Geometry: see drawing. Coordinates: mm, zero at the bounding-box minimum. A direction names the side the tool comes from. Give positions to 0.01 mm unless a question says otherwise; leave off trailing zeros. Write each loop counter-clockwise with the first axis right and the second up, starting at its lowest first coordinate (ties: lowest second). Pieces come first, ordered by that corner, then holes. Notation, with made-up numbers: (-24, 48) -> (2, 48) arc R23 ccw to (2, 56) -> close; hole circle Ø9 at (77.25, 58.25). An arc over 180 degrees is marked (long way). Use one line per item in the form item = value. Start each with the question number.
(1) Cut plane A-A, the plane y = 63.5. Output: boundary loops of the cut face in (x, z) (1 decimal).
(2) Material intervals for line 1 along X through (y, z) = (114, 19); line 2 along Y through (x, z) = (13, 23.5); line 3 along Z through (x, y) = (37, 121.5), sorted ascending. Write a range as from..to.
(3) Cut plane B-B, the plane z = 9. Output: boundary loops of the cut face in (x, y), and give its area (3 significant figures).
(4) Set-up query: the marked faces 1 and 2. Return all of +Z, -Z, +X, -X, +Y, -Y with unobstructed straight access to the full face (end or side cutting, diameter ignored); none if empty.
(5) Cut plane C-C, the plane x = 10. Output: boundary loops of the cut face in (y, z) (1 decimal).
(6) First-contact query: P1, Ø10, axis at x = 13.5, z = 21, coming from the -Y side. Flat tip, straight axial feed; report the tip coordinate or a pass-through.
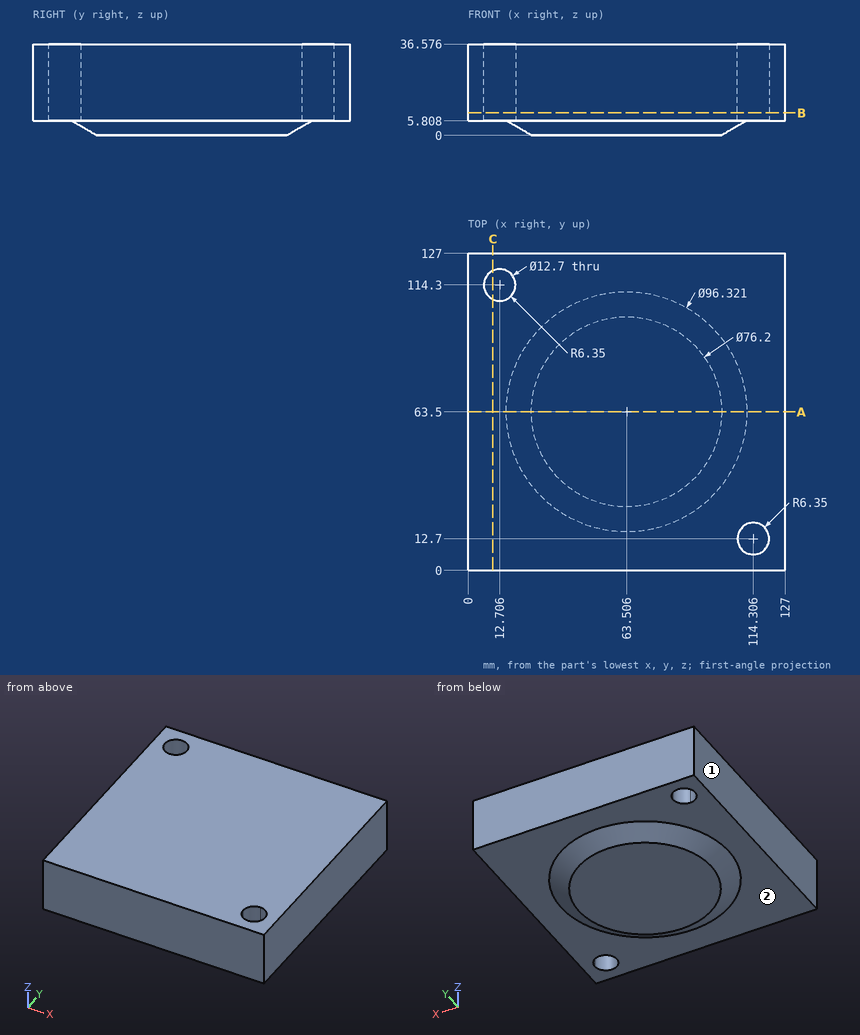
Geometry says:
q1.outline = (0, 5.8) -> (15.3, 5.8) -> (25.4, 0) -> (101.6, 0) -> (111.7, 5.8) -> (127, 5.8) -> (127, 36.6) -> (0, 36.6) -> close
q2.line_1 = 0..6.36, 19.05..127
q2.line_2 = 0..107.96, 120.64..127
q2.line_3 = 5.81..36.58
q3.outline = (0, 0) -> (127, 0) -> (127, 127) -> (0, 127) -> close; hole circle Ø12.7 at (12.71, 114.3); hole circle Ø12.7 at (114.31, 12.7)
q3.area = 15,900 mm^2
q4.face_1 = +Z, -Z, -X, +Y, -Y
q4.face_2 = -Z
q5.outline = (0, 5.8) -> (108.6, 5.8) -> (108.6, 36.6) -> (0, 36.6) -> close; (120, 5.8) -> (127, 5.8) -> (127, 36.6) -> (120, 36.6) -> close
q6.P1 = 0
